Part print with two shaded views. Sizes in mm from the minimum x, y, z corner. A direction names the side the tool comes from. Give positions to 0.01 mm unless a question says otherwise; leave off trailing zeros. Write each loop counter-clockwise with the first axis right and the second up, starting at its lowest first coordinate (ties: lowest second). Pieces come first, ordered by that corner, then holes.
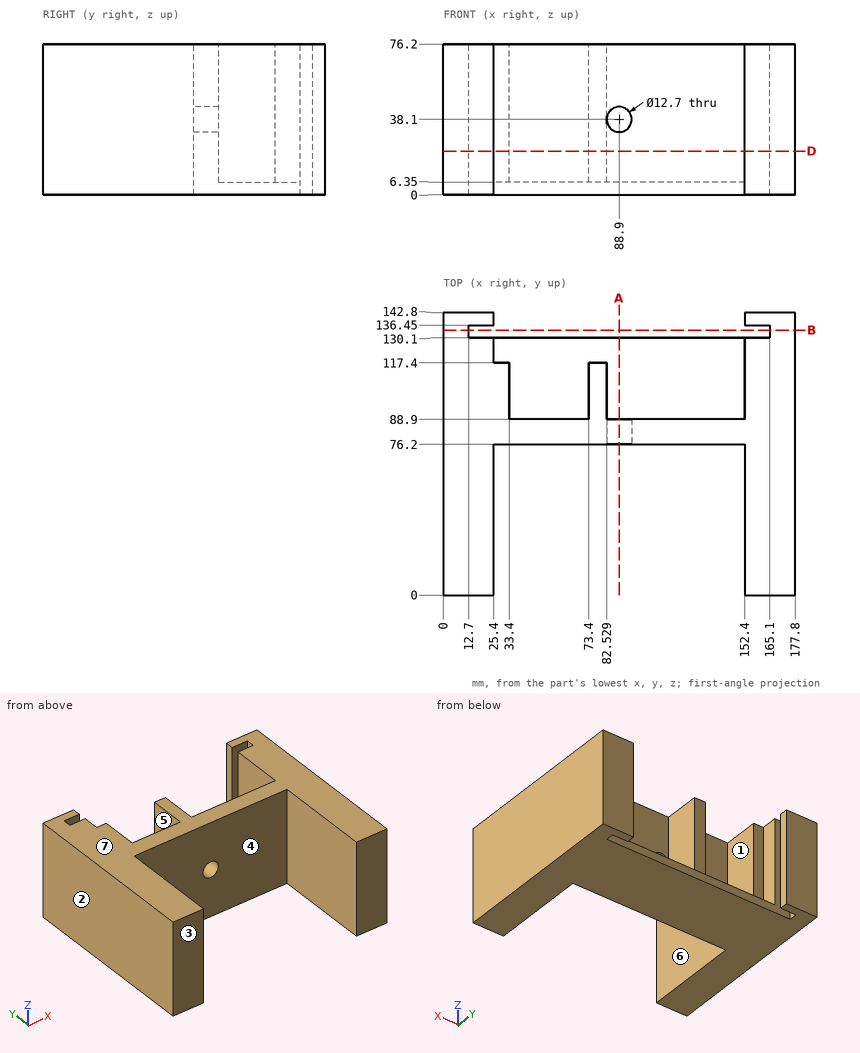
1) Flat gauge pins, fed straight in: P1, Ø21, axis at x = 105.5, z = 47, coming from the +Y side; P2, Ø1.5, axis at x = 75, z = 31.5, coming from the -Y side; P3, Ø2, axis at x = 27, z = 41, coming from the +Y side. Where does each tip first touch, or does it go through?
Check result:
P1: stops at y = 88.9
P2: stops at y = 76.2
P3: stops at y = 117.4
2) Drill centre lines: L1, parallel to X at y = 85, z = 38; L2, parallel to X at y = 40, z = 33; L3, parallel to Y at x = 21.5, z = 54. Where is each one in solid material? Low to high.
Check result:
L1: x = 0 to 82.55, 95.25 to 177.8
L2: x = 0 to 25.4, 152.4 to 177.8
L3: y = 0 to 130.1, 136.45 to 142.8
3) Saw through at D-D (z = 22). Write the cut outline in (x, y).
Check result:
outline: (0, 0) - (25.4, 0) - (25.4, 76.2) - (152.4, 76.2) - (152.4, 0) - (177.8, 0) - (177.8, 142.8) - (152.4, 142.8) - (152.4, 136.45) - (165.1, 136.45) - (165.1, 130.1) - (152.4, 130.1) - (152.4, 88.9) - (82.53, 88.9) - (82.53, 117.4) - (73.4, 117.4) - (73.4, 88.9) - (33.4, 88.9) - (33.4, 117.4) - (25.4, 117.4) - (25.4, 130.1) - (12.7, 130.1) - (12.7, 136.45) - (25.4, 136.45) - (25.4, 142.8) - (0, 142.8) - close
4) Saw through at A-A (x = 88.9). Write the cut outline in (y, z).
Check result:
outline: (76.2, 0) - (130.1, 0) - (130.1, 6.35) - (88.9, 6.35) - (88.9, 31.75) - (76.2, 31.75) - close; (76.2, 44.45) - (88.9, 44.45) - (88.9, 76.2) - (76.2, 76.2) - close
5) Saw through at B-B (y = 134). Write the cut outline in (x, z), and give its area (3 significant figures).
Check result:
outline: (0, 0) - (12.7, 0) - (12.7, 76.2) - (0, 76.2) - close; (165.1, 0) - (177.8, 0) - (177.8, 76.2) - (165.1, 76.2) - close
area: 1,940 mm2
6) Mould opens along X. For the marked faces 1, 2, 3 and 4 say: +X half, -X half, draft (parallel to the pull), parting line (faces both ways), or undercut.
Check result:
face 1: undercut
face 2: -X half
face 3: draft
face 4: undercut
7) 3-axis set-ups, long thin cutter, end or side, ignore diameter. For the marked faces 5, 6 and 7: which of +Z, -Z, +X, -X, +Y, -Y reach the whole face in a straight line?
Check result:
face 5: +Z, +Y
face 6: +Z, -Z, -Y
face 7: +Z, +X, -X, +Y, -Y
